Verification items for the finished model (mm, model axes). A direction names the side the tool comes from. Coordinates: 2 decimals unless noted, no trailing zeros. Write each loop counter-clockwise with the first axis right and the second up, starting at its lowest first coordinate (ties: lowest second). Pieces come first, ordered by that corner, then holes. Notation, with made-up numbers: M 5,-18 L 23,-18 A30 ccw 23,17 Z; hole C 39,1 d10. An arc over 180 degrees is marked long. One line per item, written item: value.
```python
from build123d import *

# Parameters (mm, degrees)
SKETCH_1_W                        = 400
SKETCH_1_H                        = 230
SM_BASE_FLANGE_1_DEPTH            = 1.5
SM_EDGE_FLANGE_1_STRIP_W          = 6.6
SM_EDGE_FLANGE_1_STRIP_H          = 1.5
SM_EDGE_FLANGE_1_STRIP_CUT_DEPTH  = 400
SM_EDGE_FLANGE_1_DEPTH            = 400
SM_EDGE_FLANGE_2_STRIP_W          = 7
SM_EDGE_FLANGE_2_STRIP_H          = 1.5
SM_EDGE_FLANGE_2_STRIP_CUT_DEPTH  = 353
SM_EDGE_FLANGE_2_RELIEF_W         = 7.75
SM_EDGE_FLANGE_2_RELIEF_H         = 0.75
SM_EDGE_FLANGE_2_RELIEF_CUT_DEPTH = 1.5
SM_EDGE_FLANGE_2_DEPTH            = 353
FILLET_1_R                        = 2
SM_START                          = -176.5
SM_EDGE_FLANGE_3_DEPTH            = 353
SM_EDGE_FLANGE_3_2_DEPTH          = 353
SM_BASE_FLANGE_1_2_DEPTH          = 1.5


# Read off the part's stored shape, not the designer's step: 边线-法兰3
# Sheet-metal steps are written as plain solids
with BuildPart() as part:
    # Sketch 1 → Sm Base Flange 1 (new body)
    with BuildSketch(Plane.XY):
        Rectangle(SKETCH_1_W, SKETCH_1_H)
    extrude(amount=-SM_BASE_FLANGE_1_DEPTH)

    # 边线-法兰1 strip (across the edge) → 边线-法兰1 strip cut (cut)
    with BuildSketch(Plane(origin=(200, -115, -1.5), x_dir=(0, 1, 0), z_dir=(-1, 0, 0))):
        with Locations((-1.5, -0.75)):
            Rectangle(SM_EDGE_FLANGE_1_STRIP_W, SM_EDGE_FLANGE_1_STRIP_H)
    extrude(amount=SM_EDGE_FLANGE_1_STRIP_CUT_DEPTH, mode=Mode.SUBTRACT)

    # 边线-法兰1 section (across the edge) → 边线-法兰1 (add)
    with BuildSketch(Plane(origin=(200, -115, -1.5), x_dir=(0, 1, 0), z_dir=(-1, 0, 0))):
        with BuildLine():
            Line((0, 0.3), (0, 23.5))
            Line((0, 23.5), (1.5, 23.5))
            Line((1.5, 23.5), (1.5, 0.3))
            ThreePointArc((1.5, 0.3), (1.587867966, 0.087867966), (1.8, 0))
            Line((1.8, 0), (1.8, -1.5))
            ThreePointArc((1.8, -1.5), (0.527207794, -0.972792206), (0, 0.3))
        make_face()
    extrude(amount=SM_EDGE_FLANGE_1_DEPTH)

    # 边线-法兰2 strip (across the edge) → 边线-法兰2 strip cut (cut)
    with BuildSketch(Plane(origin=(-176.5, -115, -25), x_dir=(0, 0, 1), z_dir=(1, 0, 0))):
        with Locations((-1.5, -0.75)):
            Rectangle(SM_EDGE_FLANGE_2_STRIP_W, SM_EDGE_FLANGE_2_STRIP_H)
    extrude(amount=SM_EDGE_FLANGE_2_STRIP_CUT_DEPTH, mode=Mode.SUBTRACT)

    # 边线-法兰2 relief (on the sheet) → 边线-法兰2 relief cut (cut)
    with BuildSketch(Plane(origin=(-176.5, -115, -23), x_dir=(0, 0, 1), z_dir=(0, -1, 0))):
        with Locations((-3.125, 0.375)):
            Rectangle(SM_EDGE_FLANGE_2_RELIEF_W, SM_EDGE_FLANGE_2_RELIEF_H)
        with Locations((-3.125, -353.375)):
            Rectangle(SM_EDGE_FLANGE_2_RELIEF_W, SM_EDGE_FLANGE_2_RELIEF_H)
    extrude(amount=-SM_EDGE_FLANGE_2_RELIEF_CUT_DEPTH, mode=Mode.SUBTRACT)

    # 边线-法兰2 section (across the edge) → 边线-法兰2 (add)
    with BuildSketch(Plane(origin=(-176.5, -115, -25), x_dir=(0, 0, 1), z_dir=(1, 0, 0))):
        with BuildLine():
            Line((0, 0.5), (0, 9.5))
            Line((0, 9.5), (1.5, 9.5))
            Line((1.5, 9.5), (1.5, 0.5))
            ThreePointArc((1.5, 0.5), (1.646446609, 0.146446609), (2, 0))
            Line((2, 0), (2, -1.5))
            ThreePointArc((2, -1.5), (0.585786438, -0.914213562), (0, 0.5))
        make_face()
    extrude(amount=SM_EDGE_FLANGE_2_DEPTH)

    # 圆角1
    fillet_1_edges = [part.edges().sort_by_distance(p)[0] for p in [
        (-200, 115, -0.75),
    ]]
    fillet(fillet_1_edges, radius=FILLET_1_R)

    # 边线-法兰3 outline → 边线-法兰3 (cut)
    with BuildSketch(Plane.YZ.offset(SM_START)):
        with BuildLine():
            ThreePointArc((-122.171572875, -25), (-122.93693974, -24.847759065), (-123.585786438, -24.414213562))
            Line((-123.585786438, -24.414213562), (-124.5, -23.5))
            Line((-124.5, -23.5), (-124.5, -25))
            Line((-124.5, -25), (-122.171572875, -25))
        make_face()
    extrude(amount=SM_EDGE_FLANGE_3_DEPTH, mode=Mode.SUBTRACT)

    # Sm Edge Flange 3 2 outline → Sm Edge Flange 3 2 (add)
    with BuildSketch(Plane.YZ.offset(SM_START)):
        with BuildLine():
            Line((-129.096194078, -18.903805922), (-124.5, -23.5))
            Line((-124.5, -23.5), (-122.171572875, -23.5))
            ThreePointArc((-122.171572875, -23.5), (-122.362914591, -23.461939766), (-122.525126266, -23.353553391))
            Line((-122.525126266, -23.353553391), (-128.035533906, -17.843145751))
            Line((-128.035533906, -17.843145751), (-129.096194078, -18.903805922))
        make_face()
    extrude(amount=SM_EDGE_FLANGE_3_2_DEPTH)

    # 草图40 → Sm Base Flange 1 2 (add)
    with BuildSketch(Plane(origin=(0, -74, -74), x_dir=(1, 0, 0), z_dir=(0, -0.7071067811865435, -0.7071067811865516))):
        Polygon((176.5, 77.9177849), (182.5, 77.9177849), (176.5, 70.124891681), align=None)
        Polygon((-176.5, 77.9177849), (-182.5, 77.9177849), (-176.5, 70.124891681), align=None)
    extrude(amount=-SM_BASE_FLANGE_1_2_DEPTH)


solid = part.part
```
Item 1: Go/stop test with flat-tipped pins: P1, Ø12, axis at x = 61.5, y = 71, coming from the -Z side; P2, Ø1, axis at x = -155.5, z = -2.5, coming from the -Y side; P3, Ø2, axis at x = -13.5, z = -5.5, coming from the +Y side; P4, Ø8, axis at y = -13, z = -9, coming from the +X side. Record where each tip stops, or that it passes through.
The answers:
P1: stops at z = -1.5
P2: stops at y = -115
P3: stops at y = -113.5
P4: passes through
Item 2: Draft check along Y on faces 3 (the face through (3, -113.5, -14)), 4 (the face through (-200, 0, -1)), 5 (the face through (3, -115, -13)). Enter one of: released by +Y, released by -Y, zero draft, split by the parting line, or undercut.
The answers:
face 3: released by +Y
face 4: zero draft
face 5: undercut
Item 3: Access from +Z, -Z, +X, -X, +Y, -Y to the whole of each face (thin tool, end or side, straight path). Record for faces 1 (the face through (200, 1, -1)), 2 (the face through (-3, 2, -1.5)).
The answers:
face 1: +Z, -Z, +X, +Y, -Y
face 2: -Z, +X, -X, +Y
Item 4: Cross-section at C-C, the plane y = 20.5. Enter the section's corners in (x, z), and give its area (3 significant figures).
The answers:
outline: M -200,-1.5 L 200,-1.5 L 200,0 L -200,0 Z
area: 600 mm²
Item 5: Scan lines: line 1 (Y direction, x = -163.5, z = -11.75); line 2 (Y direction, x = -134.5, z = -1.25); line 3 (Z direction, x = -164, y = -6). Record each from-to range of solid material in increasing order.
The answers:
line 1: y = -115 to -113.5
line 2: y = -114.91 to 115
line 3: z = -1.5 to 0
Item 6: Cross-section at B-B, the plane z = -7.5. Enter the section's corners in (x, y), and give its area (3 significant figures).
The answers:
outline: M -200,-115 L 200,-115 L 200,-113.5 L -200,-113.5 Z
area: 600 mm²
Item 7: Cross-section at A-A, the plane x = -130. Enter the section's corners in (y, z).
The answers:
outline: M -129.1,-18.9 L -123.59,-24.41 A2 ccw -122.17,-25 L -115.5,-25 A2 ccw -113.5,-23 L -113.5,-1.8 A0.3 cw -113.2,-1.5 L 115,-1.5 L 115,0 L -113.2,0 A1.8 ccw -115,-1.8 L -115,-23 A0.5 cw -115.5,-23.5 L -122.17,-23.5 A0.5 cw -122.53,-23.35 L -128.04,-17.84 Z
